```python
from build123d import *

# Parameters (mm, degrees)
SKETCH1_W           = 190.5
SKETCH1_H           = 132.08
BOSS_EXTRUDE1_DEPTH = 22.86
SKETCH2_W           = 116.84
SKETCH2_H           = 132.08
BOSS_EXTRUDE2_DEPTH = 101.6
SKETCH3_W           = 20.32
SKETCH3_H           = 101.6
BOSS_EXTRUDE3_DEPTH = 36.83
SKETCH5_W           = 55.88
SKETCH5_H           = 43.18
CUT_EXTRUDE1_DEPTH  = 46.99
SKETCH4_W           = 55.88
SKETCH4_H           = 43.18
CUT_EXTRUDE2_DEPTH  = 46.99
SKETCH6_W           = 132.08
SKETCH6_H           = 43.18
CUT_EXTRUDE3_DEPTH  = 46.99
SKETCH10_W          = 76.2
SKETCH10_H          = 132.08
CUT_EXTRUDE4_DEPTH  = 38.1
CHAMFER1_SIZE       = 36.83
CHAMFER1_SIZE2      = 101.6
FILLET1_R           = 58.42
FILLET2_R           = 38.1


# Some blends are built 0.0001 mm under size
with BuildPart() as part:
    # Sketch1 → Boss-Extrude1 (new body)
    with BuildSketch(Plane(origin=(0, 0, 0), x_dir=(1, 0, 0), z_dir=(0, 1, 0))):
        with Locations((95.25, -66.04)):
            Rectangle(SKETCH1_W, SKETCH1_H)
    extrude(amount=BOSS_EXTRUDE1_DEPTH)

    # Sketch2 → Boss-Extrude2 (add)
    with BuildSketch(Plane(origin=(0, 22.86, 0), x_dir=(1, 0, 0), z_dir=(0, 1, 0))):
        with Locations((95.25, -66.04)):
            Rectangle(SKETCH2_W, SKETCH2_H)
    extrude(amount=BOSS_EXTRUDE2_DEPTH)

    # Sketch3 → Boss-Extrude3 (add)
    with BuildSketch(Plane(origin=(153.67, 0, 0), x_dir=(0, 0, -1), z_dir=(1, 0, 0))):
        with Locations((-66.04, 73.66)):
            Rectangle(SKETCH3_W, SKETCH3_H)
    extrude(amount=BOSS_EXTRUDE3_DEPTH)

    # Sketch5 → Cut-Extrude1 (cut)
    with BuildSketch(Plane(origin=(153.67, 0, 0), x_dir=(0, 0, -1), z_dir=(1, 0, 0))):
        with Locations((-27.94, 44.45)):
            Rectangle(SKETCH5_W, SKETCH5_H)
    extrude(amount=-CUT_EXTRUDE1_DEPTH, mode=Mode.SUBTRACT)

    # Sketch4 → Cut-Extrude2 (cut)
    with BuildSketch(Plane(origin=(153.67, 0, 0), x_dir=(0, 0, -1), z_dir=(1, 0, 0))):
        with Locations((-104.14, 44.45)):
            Rectangle(SKETCH4_W, SKETCH4_H)
    extrude(amount=-CUT_EXTRUDE2_DEPTH, mode=Mode.SUBTRACT)

    # Sketch6 → Cut-Extrude3 (cut)
    with BuildSketch(Plane.ZY.offset(-36.83)):
        with Locations((66.04, 44.45)):
            Rectangle(SKETCH6_W, SKETCH6_H)
    extrude(amount=-CUT_EXTRUDE3_DEPTH, mode=Mode.SUBTRACT)

    # Sketch10 → Cut-Extrude4 (cut)
    with BuildSketch(Plane(origin=(0, 124.46, 0), x_dir=(1, 0, 0), z_dir=(0, 1, 0))):
        with Locations((95.25, -66.04)):
            Rectangle(SKETCH10_W, SKETCH10_H)
    extrude(amount=-CUT_EXTRUDE4_DEPTH, mode=Mode.SUBTRACT)

    # Chamfer1
    chamfer1_edges = [part.edges().sort_by_distance(p)[0] for p in [
        (190.5, 124.46, 66.04),
    ]]
    chamfer1_side = [part.faces().sort_by_distance(p)[0] for p in [
        (149.740639098, 124.46, 66.04),
    ]]
    chamfer(chamfer1_edges, length=CHAMFER1_SIZE, length2=CHAMFER1_SIZE2, reference=chamfer1_side[0])

    # Fillet1
    # the kernel refuses this fillet: 58.42 mm, written as the material it takes off along each edge
    with BuildSketch(Plane(origin=(36.83, 66.04, 275.307343322), x_dir=(0, 1, 0), z_dir=(0, 0, -1))) as fillet1_piece_1:
        with BuildLine():
            CenterArc((57.290937329, 58.42), FILLET1_R, 191.282824288, 78.717175712)
            Line((0, 46.99), (-1.145818747, 46.7614))
            ThreePointArc((-1.145818747, 46.7614), (-1.1684, 23.495), (-1.1684, 0))
            Line((-1.1684, 0), (0, -1.1684))
            Line((0, -1.1684), (57.290937329, -1.1684))
            Line((57.290937329, -1.1684), (57.290937329, 0))
        make_face()
    extrude(amount=418.534686643, mode=Mode.SUBTRACT)
    with BuildSketch(Plane(origin=(153.67, 66.04, -143.227343322), x_dir=(-1, 0, 0), z_dir=(0, 0, 1))) as fillet1_piece_2:
        with BuildLine():
            CenterArc((58.42, -57.290937329), FILLET1_R, 101.282824288, 78.717175712)
            Line((0, -57.290937329), (-1.1684, -57.290937329))
            Line((-1.1684, -57.290937329), (-1.1684, 0))
            Line((-1.1684, 0), (0, 1.1684))
            ThreePointArc((0, 1.1684), (23.495, 1.1684), (46.7614, 1.145818747))
            Line((46.7614, 1.145818747), (46.99, 0))
        make_face()
    extrude(amount=199.107343322, mode=Mode.SUBTRACT)
    with BuildSketch(Plane(origin=(153.67, 66.04, -143.227343322), x_dir=(-1, 0, 0), z_dir=(0, 0, 1))) as fillet1_piece_3_section:
        with BuildLine():
            CenterArc((58.42, -57.290937329), FILLET1_R, 101.282824288, 78.717175712)
            Line((0, -57.290937329), (-1.1684, -57.290937329))
            Line((-1.1684, -57.290937329), (-1.1684, 0))
            Line((-1.1684, 0), (0, 1.1684))
            ThreePointArc((0, 1.1684), (23.495, 1.1684), (46.7614, 1.145818747))
            Line((46.7614, 1.145818747), (46.99, 0))
        make_face()
    fillet1_piece_3 = extrude(amount=342.334686643, mode=Mode.PRIVATE)
    fillet1_piece_3 = split(fillet1_piece_3, bisect_by=Plane(origin=(141.963702204, 79.396824985, 76.2), z_dir=(0, 0, 1)), keep=Keep.TOP, mode=Mode.PRIVATE)
    add(fillet1_piece_3, mode=Mode.SUBTRACT)
    with BuildSketch(Plane(origin=(153.67, 66.04, 275.307343322), x_dir=(0, 1, 0), z_dir=(0, 0, -1))) as fillet1_piece_4:
        with BuildLine():
            CenterArc((57.290937329, -58.42), FILLET1_R, 90, 78.717175712)
            Line((0, -46.99), (-1.145818747, -46.7614))
            ThreePointArc((-1.145818747, -46.7614), (-1.1684, -23.495), (-1.1684, 0))
            Line((-1.1684, 0), (0, 1.1684))
            Line((0, 1.1684), (57.290937329, 1.1684))
            Line((57.290937329, 1.1684), (57.290937329, 0))
        make_face()
    extrude(amount=199.107343322, mode=Mode.SUBTRACT)
    with BuildSketch(Plane(origin=(153.67, 66.04, 275.307343322), x_dir=(0, 1, 0), z_dir=(0, 0, -1))) as fillet1_piece_5_section:
        with BuildLine():
            CenterArc((57.290937329, -58.42), FILLET1_R, 90, 78.717175712)
            Line((0, -46.99), (-1.145818747, -46.7614))
            ThreePointArc((-1.145818747, -46.7614), (-1.1684, -23.495), (-1.1684, 0))
            Line((-1.1684, 0), (0, 1.1684))
            Line((0, 1.1684), (57.290937329, 1.1684))
            Line((57.290937329, 1.1684), (57.290937329, 0))
        make_face()
    fillet1_piece_5 = extrude(amount=342.334686643, mode=Mode.PRIVATE)
    fillet1_piece_5 = split(fillet1_piece_5, bisect_by=Plane(origin=(141.963702204, 79.396824985, 55.88), z_dir=(0, 0, -1)), keep=Keep.TOP, mode=Mode.PRIVATE)
    add(fillet1_piece_5, mode=Mode.SUBTRACT)

    # Fillet2
    fillet2_edges = [part.edges().sort_by_distance(p)[0] for p in [
        (133.35, 86.36, 66.04),
        (57.15, 86.36, 66.04),
    ]]
    fillet(fillet2_edges, radius=FILLET2_R - 0.0001)  # a hair under: the kernel refuses the full size


solid = part.part
```
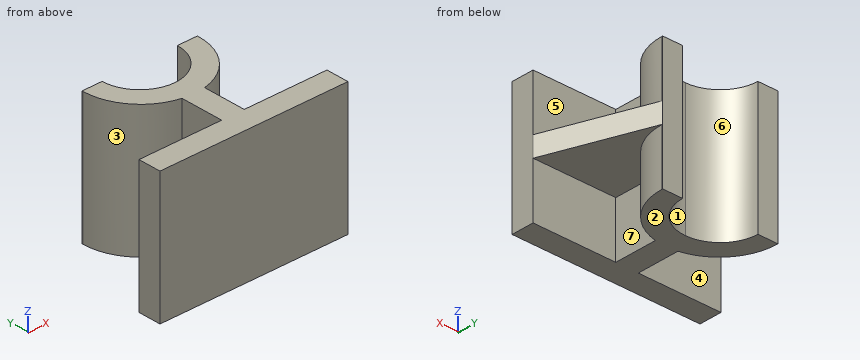
Here's how the part is built. I have some questions about the finished solid (model axes, mm). Face numbers are marked on the shaded views. A direction names the side the tool comes from. Give positions to 0.01 mm unless a question says otherwise; leave off trailing zeros. Write each loop counter-clockwise with the first axis right and the second up, starting at its lowest first coordinate (ties: lowest second). Pieces come first, ordered by that corner, then holes.
(1) Imagine slicing it at B-B, the plane x = 68.5. Write out the boundary of the cut face in (y, z), and give its area (3 significant figures).
Output values:
outline: (0, 0) - (22.86, 0) - (22.86, 132.08) - (0, 132.08) - close; (71.4, 0) - (97.33, 0) - (97.33, 132.08) - (71.4, 132.08) - close
area: 6,440 mm2
(2) Imagine slicing it at D-D, the plane y = 60. Write out the boundary of the cut face in (x, z).
Output values:
outline: (83.82, 0) - (106.68, 0) - (106.68, 55.88) - (177.04, 55.88) - (177.04, 76.2) - (106.68, 76.2) - (106.68, 132.08) - (83.82, 132.08) - close
(3) Thinking about a two-plate mould opening in Y: for the marked faces 1, 2 and 3, which applies, pulls with the +Y half, pulls with the -Y half, needs draft (parallel to the pull), parting line crosses it, or undercut?
Output values:
face 1: pulls with the +Y half
face 2: needs draft
face 3: undercut
(4) Imagine slicing it at C-C, the plane y = 117.5. Write out the boundary of the cut face in (x, z), and give its area (3 significant figures).
Output values:
outline: (37.12, 0) - (57.79, 0) - (57.79, 132.08) - (37.12, 132.08) - close; (132.71, 0) - (153.38, 0) - (153.38, 55.88) - (156.19, 55.88) - (156.19, 76.2) - (153.38, 76.2) - (153.38, 132.08) - (132.71, 132.08) - close
area: 5,520 mm2
(5) Will these pins go through, and if not, where does the flat tip stop? pin 1 (1 mm diameter, centred on y = 47, z = 41.5, fed in from -X); pin 2 (25 mm diameter, centred on x = 165.5, y = 88, fed in from -Z); pin 3 (12 mm diameter, centred on y = 90.5, z = 57, fed in from +X).
Output values:
pin 1: stops at x = 83.82
pin 2: stops at z = 55.88
pin 3: stops at x = 168.16
(6) On a 3-axis mill with a long thin cutter (end or side, diameter ignored), from which of +Z, -Z, +X, -X, +Y, -Y can I reach the whole of each face in a straight line? I mean the marked faces 4, 5, 6 and 7. Say none if no direction works.
Output values:
face 4: +Z, -Z, -X
face 5: +Z, +X
face 6: +Z, -Z, +Y
face 7: -Z, +X
(7) If I drill on L1, parallel to Y at x = 8.5, z = 90; L2, parallel to Z at x = 110.5, y = 35.5; L3, parallel to X at y = 36.5, z = 121, over which ranges is the centre line in solid material (lowest first)?
Output values:
L1: y = 0 to 22.86
L2: z = 55.88 to 76.2
L3: x = 83.82 to 106.68
